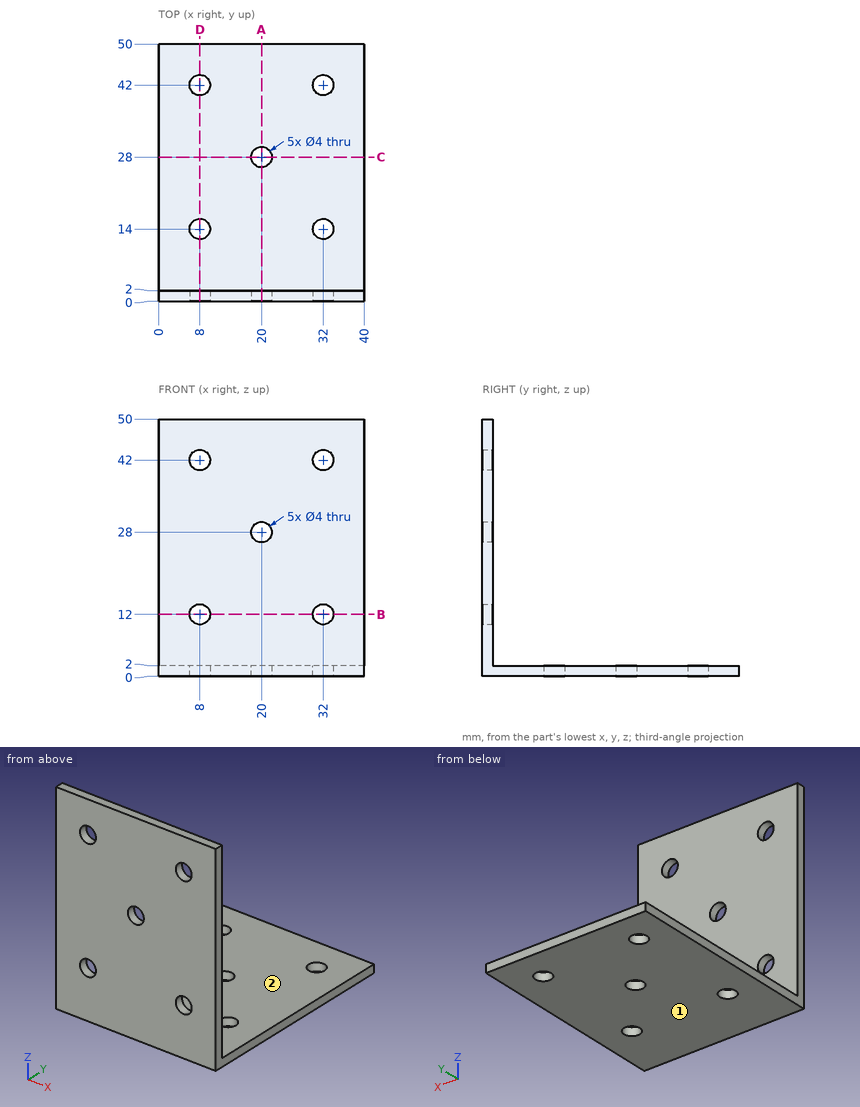
Geometry check sheet. Reference: drawing and pictorial views, mm from the part's lowest x, y, z. A direction names the side the tool comes from. Give positions to 0.01 mm unless a question says otherwise; leave off trailing zeros. Write each loop counter-clockwise with the first axis right and the second up, starting at its lowest first coordinate (ties: lowest second). Pieces come first, ordered by that corner, then holes. Notation, with made-up numbers: M 24.25,15 L 56.25,15 A31 cw 56.25,51 Z; hole C -18.5,-22.5 d3. An arc over 180 degrees is marked long. Answer as CSV lines item,"result". Start each with the question number.
Q1. Section check C-C, the plane y = 28. Record the cut outline in (x, z).
Q2. Section check B-B, the plane z = 12. Record the cut outline in (x, y).
Q3. Tool access check on the marked faces 1 and 2. Record the directions out of +Z, -Z, +X, -X, +Y, -Y that give a thin tool (end or side, any length) a straight path to the whole face; none if there is none.
Q4. Material ranges on L1, parallel to X at y = 1.55, z = 42; L2, parallel to Y at x = 8, z = 1.5; L3, parallel to Z at x = 16, y = 26, recorded low to high.
Q5. Section check D-D, the plane x = 8. Record the cut outline in (y, z), then the cut area to 3 significant figures.
Q6. Section check A-A, the plane x = 20. Record the cut outline in (y, z), then the cut area to 3 significant figures.
Q7. Go/stop test with flat-tipped pins: pin 1 (6.5 mm diameter, centred on x = 32, y = 14, fed in from +Z); pin 2 (6.5 mm diameter, centred on x = 32, z = 12, fed in from +Y). Record where each tip stops, or that it passes through.
Geometry says:
1,outline,"M 0,0 L 18,0 L 18,2 L 0,2 Z; M 22,0 L 40,0 L 40,2 L 22,2 Z"
2,outline,"M 0,0 L 6,0 L 6,2 L 0,2 Z; M 10,0 L 30,0 L 30,2 L 10,2 Z; M 34,0 L 40,0 L 40,2 L 34,2 Z"
3,face 1,"-Z, +X, -X, +Y, -Y"
3,face 2,"+Z, +X, -X, +Y"
4,L1,"0 to 6, 10 to 30, 34 to 40"
4,L2,"0 to 12, 16 to 40, 44 to 50"
4,L3,"0 to 2"
5,outline,"M 0,0 L 12,0 L 12,2 L 2,2 L 2,10 L 0,10 Z; M 0,14 L 2,14 L 2,40 L 0,40 Z; M 0,44 L 2,44 L 2,50 L 0,50 Z; M 16,0 L 40,0 L 40,2 L 16,2 Z; M 44,0 L 50,0 L 50,2 L 44,2 Z"
5,area,"164 mm^2"
6,outline,"M 0,0 L 26,0 L 26,2 L 2,2 L 2,26 L 0,26 Z; M 0,30 L 2,30 L 2,50 L 0,50 Z; M 30,0 L 50,0 L 50,2 L 30,2 Z"
6,area,"180 mm^2"
7,pin 1,"z = 2"
7,pin 2,"y = 2"
